from build123d import *

# Parameters (mm, degrees)
BOSS_EXTRUDE1_DEPTH  = 10
SKETCH2_R            = 25
BOSS_EXTRUDE2_DEPTH  = 48
SKETCH3_R            = 16
CUT_EXTRUDE1_DEPTH   = 59
BOSS_EXTRUDE3_DEPTH  = 25
BOSS_EXTRUDE5_DEPTH  = 10
SKETCH6_R            = 20
BOSS_EXTRUDE6_DEPTH  = 8
SKETCH7_R            = 10
CUT_EXTRUDE2_DEPTH   = 16
FILLET1_R            = 25
FILLET1_OF_MIRROR1_R = 25
CUT_EXTRUDE3_REACH   = 12
SKETCH8_R            = 5


with BuildPart() as part:
    # Sketch1 → Boss-Extrude1 (new body)
    with BuildSketch(Plane(origin=(0, 0, 0), x_dir=(1, 0, 0), z_dir=(0, 1, 0))):
        with BuildLine():
            Line((-45, 28), (45, 28))
            Line((45, 28), (45, 6))
            ThreePointArc((45, 6), (48.514718626, -2.485281374), (57, -6))
            ThreePointArc((57, -6), (65.485281374, -9.514718626), (69, -18))
            Line((69, -18), (69, -50))
            Line((69, -50), (75, -50))
            Line((75, -50), (75, -60))
            Line((75, -60), (35, -60))
            Line((35, -60), (35, -35))
            Line((35, -35), (-35, -35))
            Line((-35, -35), (-35, -60))
            Line((-35, -60), (-75, -60))
            Line((-75, -60), (-75, -50))
            Line((-75, -50), (-69, -50))
            Line((-69, -50), (-69, -18))
            ThreePointArc((-69, -18), (-65.485281374, -9.514718626), (-57, -6))
            ThreePointArc((-57, -6), (-48.514718626, -2.485281374), (-45, 6))
            Line((-45, 6), (-45, 28))
        make_face()
    extrude(amount=BOSS_EXTRUDE1_DEPTH)

    # Sketch2 → Boss-Extrude2 (add)
    with BuildSketch(Plane(origin=(0, 10, 0), x_dir=(1, 0, 0), z_dir=(0, 1, 0))):
        with Locations(Location((0, 0, 0), (0, 0, 270))):  # turned: the seam where the file's is
            Circle(SKETCH2_R)
    extrude(amount=BOSS_EXTRUDE2_DEPTH)

    # Sketch3 → Cut-Extrude1 (cut, through all)
    with BuildSketch(Plane(origin=(0, 58, 0), x_dir=(1, 0, 0), z_dir=(0, 1, 0))):
        with Locations(Location((0, 0, 0), (0, 0, 270))):  # turned: the seam where the file's is
            Circle(SKETCH3_R)
    extrude(amount=-CUT_EXTRUDE1_DEPTH, mode=Mode.SUBTRACT)

    # Sketch4 → Boss-Extrude3 (add)
    with BuildSketch(Plane(origin=(0, 10, 0), x_dir=(1, 0, 0), z_dir=(0, 1, 0))):
        with BuildLine():
            Line((-25, 0), (-25, -22))
            ThreePointArc((-25, -22), (-25.878679656, -24.121320344), (-28, -25))
            Line((-28, -25), (-33, -25))
            ThreePointArc((-33, -25), (-41.485281374, -28.514718626), (-45, -37))
            Line((-45, -37), (-45, -47))
            ThreePointArc((-45, -47), (-45.878679656, -49.121320344), (-48, -50))
            Line((-48, -50), (-75, -50))
            Line((-75, -50), (-75, -60))
            Line((-75, -60), (-35, -60))
            Line((-35, -60), (-35, -35))
            Line((-35, -35), (35, -35))
            Line((35, -35), (35, -60))
            Line((35, -60), (75, -60))
            Line((75, -60), (75, -50))
            Line((75, -50), (48, -50))
            ThreePointArc((48, -50), (45.878679656, -49.121320344), (45, -47))
            Line((45, -47), (45, -37))
            ThreePointArc((45, -37), (41.485281374, -28.514718626), (33, -25))
            Line((33, -25), (28, -25))
            ThreePointArc((28, -25), (25.878679656, -24.121320344), (25, -22))
            Line((25, -22), (25, 0))
            ThreePointArc((25, 0), (0, -25), (-25, 0))
        make_face()
    extrude(amount=BOSS_EXTRUDE3_DEPTH)

    # Sketch5 → Boss-Extrude5 (add)
    with BuildSketch(Plane.ZY.offset(45)):
        with BuildLine():
            Line((-28, 0), (-19.859709814, -68.364725376))
            ThreePointArc((-19.859709814, -68.364725376), (-1.119802535, -85.96862645), (19.470806475, -70.570305811))
            Line((19.470806475, -70.570305811), (36.035496755, 0))
            Line((36.035496755, 0), (-28, 0))
        make_face()
    boss_extrude5 = extrude(amount=-BOSS_EXTRUDE5_DEPTH)

    # Sketch6 → Boss-Extrude6 (add, symmetric)
    with BuildSketch(Plane.ZY.offset(40)):
        with Locations((0, -66)):
            Circle(SKETCH6_R)
    boss_extrude6 = extrude(amount=BOSS_EXTRUDE6_DEPTH, both=True)

    # Sketch7 → Cut-Extrude2 (cut)
    with BuildSketch(Plane.ZY.offset(48)):
        with Locations((0, -66)):
            Circle(SKETCH7_R)
    cut_extrude2 = extrude(amount=-CUT_EXTRUDE2_DEPTH, mode=Mode.SUBTRACT)

    # Fillet1
    fillet1_edges = [part.edges().sort_by_distance(p)[0] for p in [
        (-40, 0, 36.035496755),
    ]]
    fillet(fillet1_edges, radius=FILLET1_R)

    # Mirror1: Boss-Extrude5, Boss-Extrude6, Cut-Extrude2 across plane
    add(boss_extrude5.mirror(Plane(origin=(0, 0, 0), x_dir=(0, 0, 1), z_dir=(1, 0, 0))))
    add(boss_extrude6.mirror(Plane(origin=(0, 0, 0), x_dir=(0, 0, 1), z_dir=(1, 0, 0))))
    add(cut_extrude2.mirror(Plane(origin=(0, 0, 0), x_dir=(0, 0, 1), z_dir=(1, 0, 0))), mode=Mode.SUBTRACT)

    # Fillet1 of Mirror1
    fillet1_of_mirror1_edges = [part.edges().sort_by_distance(p)[0] for p in [
        (40, 0, 36.035496755),
    ]]
    fillet(fillet1_of_mirror1_edges, radius=FILLET1_OF_MIRROR1_R)

    # Sketch8 → Cut-Extrude3 (cut, up to next)
    with BuildSketch(Plane(origin=(0, 0, 50), x_dir=(-1, 0, 0), z_dir=(0, 0, -1)), mode=Mode.PRIVATE) as cut_extrude3_sk1:
        with Locations((-60, 20)):
            Circle(SKETCH8_R)
    cut_extrude3_tool1 = extrude(cut_extrude3_sk1.sketch, amount=-CUT_EXTRUDE3_REACH, mode=Mode.PRIVATE) & part.part
    add(cut_extrude3_tool1.solids().sort_by_distance((60, 20, 50))[0], mode=Mode.SUBTRACT)
    # Sketch8 → Cut-Extrude3 (cut, up to next)
    with BuildSketch(Plane(origin=(0, 0, 50), x_dir=(-1, 0, 0), z_dir=(0, 0, -1)), mode=Mode.PRIVATE) as cut_extrude3_sk2:
        with Locations((60, 20)):
            Circle(SKETCH8_R)
    cut_extrude3_tool2 = extrude(cut_extrude3_sk2.sketch, amount=-CUT_EXTRUDE3_REACH, mode=Mode.PRIVATE) & part.part
    add(cut_extrude3_tool2.solids().sort_by_distance((-60, 20, 50))[0], mode=Mode.SUBTRACT)


solid = part.part
Source: CAD feature listing. Evaluate the final solid. Frame: model axes, mm. A direction names the side the tool comes from. Round coordinates to 2 decimals unless told otherwise and drop trailing zeros. Loops run counter-clockwise (first coordinate to the right, second up) from the corner with the lowest first, then second, coordinate; pieces in that order, holes last. Notation, with made-up numbers: (17.25, 75.5) - (50.25, 75.5) arc R27 ccw to (50.25, 98.5) - close; hole circle Ø6 at (15, -34.75). An arc over 180 degrees is marked (long way). Write item = value, one per line. Start each with the question number.
(1) Pull-direction query (X, two-part tool) for faces 4 (the face through (55, 17, 60)), 5 (the face through (-69, 5, 34)), 6 (the face through (0, 17, 35)); classes: +X half, -X half, draft (parallel to the pull), parting line (faces both ways), or undercut.
(2) Section query C-C, the plane z = 43.5. Output: boundary loops of the cut face in (x, y).
(3) Set-up query: faces 1 (the face through (1.099, 38.997, -24.976)), 2 (the face through (32, 10, 10)), 3 (the face through (41.58, 22.32, 28.61)). Return all of +Z, -Z, +X, -X, +Y, -Y with unobstructed straight access to the full face (end or side cutting, diameter ignored); none if empty.
(4) Pin query (flat end, axial travel): pin 1 (1.5 mm diameter, centred on x = 31.5, y = 20, fed in from -Z); pin 2 (1 mm diameter, centred on x = 7.5, y = 7.5, fed in from +Z); pin 3 (24 mm diameter, centred on y = 26.5, z = 14.5, fed in from +X); pin 4 (6 mm diameter, centred on x = -60, y = 20, fed in from +Z). Return the tip coordinate at first contact, or that it passes through.
(5) Section query A-A, the plane y = 20. State how many separate pieces and enclosed holes the cut face has, plus the area to 3 significant figures.
(6) Section query B-B, the plane x = 0. Output: boundary loops of the cut face in (y, z), plus the area to 3 significant figures.
(7) Ray query, line 1 along X through (y, z) = (-15.5, -10.5); line 2 along Y through (x, z) = (60, 55.25); line 3 along Y through (x, z) = (42, 0). Return the intervals inside material, ascending. Write a range as from..to.
Conclusion:
q1.face_4 = draft
q1.face_5 = -X half
q1.face_6 = undercut
q2.outline = (-69, 0) - (-45, 0) - (-45, -3.26) - (-35, -3.26) - (-35, 35) - (-45, 35) - (-45, 10) - (-69, 10) - close; (35, -3.26) - (45, -3.26) - (45, 0) - (69, 0) - (69, 10) - (45, 10) - (45, 35) - (35, 35) - close
q3.face_1 = +Y
q3.face_2 = -Z, +Y
q3.face_3 = -Z, +X, +Y
q4.pin_1 = 25
q4.pin_2 = 35
q4.pin_3 = 38.81
q4.pin_4 = through
q5.separate_pieces = 3
q5.enclosed_holes = 1
q5.area = 3,170 mm2
q6.outline = (0, -28) - (10, -28) - (10, -25) - (58, -25) - (58, -16) - (0, -16) - close; (0, 16) - (58, 16) - (58, 25) - (35, 25) - (35, 35) - (0, 35) - close
q6.area = 1,420 mm2
q7.line_1 = -45..-35, 35..45
q7.line_2 = 0..15, 25..35
q7.line_3 = -86..-76, -56..10
